Could you check a few things on this model? Use its own coordinates, in mm. Face numbers are marked on the shaded views. A direction names the side the tool comes from. Round coordinates to 2 decimals unless told otherwise and drop trailing zeros. Write each loop counter-clockwise with the first axis right and the second up, starting at its lowest first coordinate (ties: lowest second). Pieces come first, ordered by that corner, then holes. Notation, with made-up numbers: (38.25, 87) -> (91.25, 87) arc R24 ccw to (91.25, 102) -> close; hole circle Ø11 at (-16, 45.5). An arc over 180 degrees is marked (long way). Return JSON: item names as keys, results as strings.
from build123d import *

# Parameters (mm, degrees)
F1_DEPTH = 5
F2_DEPTH = 40
F3_DEPTH = 30


with BuildPart() as f1:
    # F0 (on Front) → F1 (new body)
    with BuildSketch(Plane.XZ):
        with BuildLine():
            Line((-22.0933434024, -7.5), (-27.3651991933, -7.5))
            ThreePointArc((-27.3651991933, -7.5), (-24.7292712978, -7.9784699581), (-22.0933434024, -7.5))
        make_face()
        with BuildLine():
            Line((27.7367906295, -7.5), (22.4649348386, -7.5))
            ThreePointArc((22.4649348386, -7.5), (25.1008627341, -7.9784699581), (27.7367906295, -7.5))
        make_face()
        with BuildLine():
            Line((32.5, -7.5), (32.5, -1.7043442256))
            ThreePointArc((32.5, -1.7043442256), (30.8950874158, -5.2405031728), (27.7367906295, -7.5))
            Line((27.7367906295, -7.5), (32.5, -7.5))
        make_face()
        with BuildLine():
            ThreePointArc((32.6008627341, -0.4784699581), (32.5756045187, 0.1365383775), (32.5, 0.7474043095))
            Line((32.5, 0.7474043095), (32.5, -1.7043442256))
            ThreePointArc((32.5, -1.7043442256), (32.5756045187, -1.0934782936), (32.6008627341, -0.4784699581))
        make_face()
        with BuildLine():
            Line((32.5, 7.5), (6.6143782777, 7.5))
            ThreePointArc((6.6143782777, 7.5), (9.1143782777, 4.1143782777), (10, 0))
            ThreePointArc((10, 0), (9.1143782777, -4.1143782777), (6.6143782777, -7.5))
            Line((6.6143782777, -7.5), (22.4649348386, -7.5))
            ThreePointArc((22.4649348386, -7.5), (20.3388295194, 5.3157547236), (32.5, 0.7474043095))
            Line((32.5, 0.7474043095), (32.5, 7.5))
        make_face()
        with BuildLine():
            Line((6.6143782777, 7.5), (-6.6143782777, 7.5))
            ThreePointArc((-6.6143782777, 7.5), (-10, 0), (-6.6143782777, -7.5))
            Line((-6.6143782777, -7.5), (-2.2328131871, -7.5))
            ThreePointArc((-2.2328131871, -7.5), (-4.1794324094, 5.698071659), (7.6857957181, -0.4006809507))
            ThreePointArc((7.6857957181, -0.4006809507), (6.2845483278, -4.7659090782), (2.6044046233, -7.5))
            Line((2.6044046233, -7.5), (6.6143782777, -7.5))
            ThreePointArc((6.6143782777, -7.5), (9.1143782777, -4.1143782777), (10, 0))
            ThreePointArc((10, 0), (9.1143782777, 4.1143782777), (6.6143782777, 7.5))
        make_face()
        with BuildLine():
            Line((-6.6143782777, 7.5), (-32.5, 7.5))
            Line((-32.5, 7.5), (-32.5, -7.5))
            Line((-32.5, -7.5), (-27.3651991933, -7.5))
            ThreePointArc((-27.3651991933, -7.5), (-29.0001342542, 5.6867331698), (-17.2292712978, -0.4784699581))
            ThreePointArc((-17.2292712978, -0.4784699581), (-18.56406817, -4.7493329144), (-22.0933434024, -7.5))
            Line((-22.0933434024, -7.5), (-6.6143782777, -7.5))
            ThreePointArc((-6.6143782777, -7.5), (-10, 0), (-6.6143782777, 7.5))
        make_face()
        with BuildLine():
            ThreePointArc((7.6857957181, -0.4006809507), (-4.1794324094, 5.698071659), (-2.2328131871, -7.5))
            Line((-2.2328131871, -7.5), (2.6044046233, -7.5))
            ThreePointArc((2.6044046233, -7.5), (6.2845483278, -4.7659090782), (7.6857957181, -0.4006809507))
        make_face()
        with BuildLine():
            ThreePointArc((-17.2292712978, -0.4784699581), (-29.0001342542, 5.6867331698), (-27.3651991933, -7.5))
            Line((-27.3651991933, -7.5), (-22.0933434024, -7.5))
            ThreePointArc((-22.0933434024, -7.5), (-18.56406817, -4.7493329144), (-17.2292712978, -0.4784699581))
        make_face()
        with BuildLine():
            Line((32.5, -1.7043442256), (32.5, 0.7474043095))
            ThreePointArc((32.5, 0.7474043095), (20.3388295194, 5.3157547236), (22.4649348386, -7.5))
            Line((22.4649348386, -7.5), (27.7367906295, -7.5))
            ThreePointArc((27.7367906295, -7.5), (30.8950874158, -5.2405031728), (32.5, -1.7043442256))
        make_face()
    extrude(amount=F1_DEPTH)

    # F0 (on Front) → F2 (join)
    with BuildSketch(Plane.XZ):
        with BuildLine():
            ThreePointArc((7.6857957181, -0.4006809507), (-4.1794324094, 5.698071659), (-2.2328131871, -7.5))
            Line((-2.2328131871, -7.5), (2.6044046233, -7.5))
            ThreePointArc((2.6044046233, -7.5), (6.2845483278, -4.7659090782), (7.6857957181, -0.4006809507))
        make_face()
        with BuildLine():
            ThreePointArc((6.6143782777, 7.5), (0, 10), (-6.6143782777, 7.5))
            Line((-6.6143782777, 7.5), (6.6143782777, 7.5))
        make_face()
        with BuildLine():
            Line((-2.2328131871, -7.5), (-6.6143782777, -7.5))
            ThreePointArc((-6.6143782777, -7.5), (0, -10), (6.6143782777, -7.5))
            Line((6.6143782777, -7.5), (2.6044046233, -7.5))
            ThreePointArc((2.6044046233, -7.5), (0.1857957181, -7.9006809507), (-2.2328131871, -7.5))
        make_face()
        with BuildLine():
            Line((6.6143782777, 7.5), (-6.6143782777, 7.5))
            ThreePointArc((-6.6143782777, 7.5), (-10, 0), (-6.6143782777, -7.5))
            Line((-6.6143782777, -7.5), (-2.2328131871, -7.5))
            ThreePointArc((-2.2328131871, -7.5), (-4.1794324094, 5.698071659), (7.6857957181, -0.4006809507))
            ThreePointArc((7.6857957181, -0.4006809507), (6.2845483278, -4.7659090782), (2.6044046233, -7.5))
            Line((2.6044046233, -7.5), (6.6143782777, -7.5))
            ThreePointArc((6.6143782777, -7.5), (9.1143782777, -4.1143782777), (10, 0))
            ThreePointArc((10, 0), (9.1143782777, 4.1143782777), (6.6143782777, 7.5))
        make_face()
    extrude(amount=F2_DEPTH)

    # F0 (on Front) → F3 (join)
    with BuildSketch(Plane.XZ):
        with BuildLine():
            Line((32.5, -1.7043442256), (32.5, 0.7474043095))
            ThreePointArc((32.5, 0.7474043095), (20.3388295194, 5.3157547236), (22.4649348386, -7.5))
            Line((22.4649348386, -7.5), (27.7367906295, -7.5))
            ThreePointArc((27.7367906295, -7.5), (30.8950874158, -5.2405031728), (32.5, -1.7043442256))
        make_face()
        with BuildLine():
            ThreePointArc((-17.2292712978, -0.4784699581), (-29.0001342542, 5.6867331698), (-27.3651991933, -7.5))
            Line((-27.3651991933, -7.5), (-22.0933434024, -7.5))
            ThreePointArc((-22.0933434024, -7.5), (-18.56406817, -4.7493329144), (-17.2292712978, -0.4784699581))
        make_face()
        with BuildLine():
            ThreePointArc((7.6857957181, -0.4006809507), (-4.1794324094, 5.698071659), (-2.2328131871, -7.5))
            Line((-2.2328131871, -7.5), (2.6044046233, -7.5))
            ThreePointArc((2.6044046233, -7.5), (6.2845483278, -4.7659090782), (7.6857957181, -0.4006809507))
        make_face()
    extrude(amount=-F3_DEPTH)


solid = f1.part
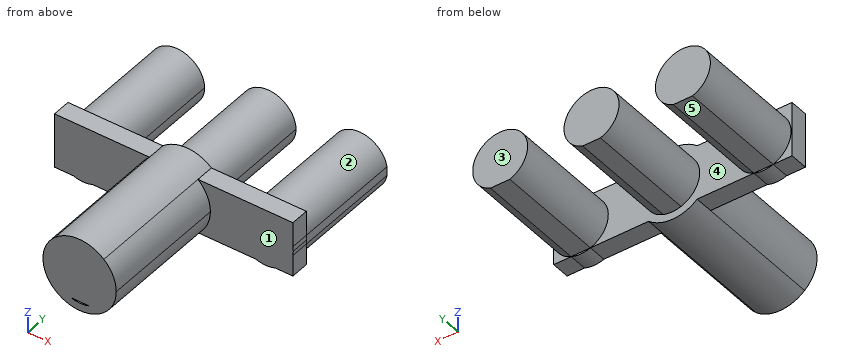
1) I want a section at A-A, the plane y = 4. Please give me the cut outline in (x, z), and give its area (3 significant figures).
Return value:
{"outline": "(-27.37, -7.5) -> (-22.09, -7.5) arc R7.5 ccw (long way) to start; (-2.23, -7.5) -> (2.6, -7.5) arc R7.5 ccw (long way) to start; (22.46, -7.5) -> (27.74, -7.5) arc R7.5 ccw to (32.5, -1.7) -> (32.5, 0.75) arc R7.5 ccw (long way) to start", "area": "525 mm²"}
2) Thinking about a two-plate mould opening in X: for the marked faces 1 and 2, which applies, pulls with the +X half, pulls with the -X half, needs draft (parallel to the pull), parting line crosses it, or undercut?
Return value:
{"face 1": "needs draft", "face 2": "undercut"}
3) Will these pins go through, and if not, where does the flat tip stop? pin 1 Ø1.5 at (x, y) = (15.5, -1.5) entering from +Z; pin 2 Ø2 at (y, z) = (13.5, -0.5) entering from +X; pin 3 Ø5 at (x, y) = (-7, -2) entering from -Z; pin 4 Ø10 at (x, z) = (10, 3) entering from -Y.
Return value:
{"pin 1": "z = 7.5", "pin 2": "x = 32.5", "pin 3": "z = -8.93", "pin 4": "y = -40"}
4) I want a section at D-D, the plane z = 4. Please give me the cut outline in (x, y).
Return value:
{"outline": "(-32.5, -5) -> (-9.17, -5) -> (-9.17, -40) -> (9.17, -40) -> (9.17, -5) -> (32.5, -5) -> (32.5, 0) -> (31.12, 0) -> (31.12, 30) -> (19.08, 30) -> (19.08, 0) -> (6.26, 0) -> (6.26, 30) -> (-5.89, 30) -> (-5.89, 0) -> (-18.71, 0) -> (-18.71, 30) -> (-30.75, 30) -> (-30.75, 0) -> (-32.5, 0) -> close"}
5) I want a section at C-C, the plane z = -2.5. Please give me the cut outline in (x, y).
Return value:
{"outline": "(-32.5, -5) -> (-9.68, -5) -> (-9.68, -40) -> (9.68, -40) -> (9.68, -5) -> (32.5, -5) -> (32.5, 0) -> (32.32, 0) -> (32.32, 30) -> (17.88, 30) -> (17.88, 0) -> (7.39, 0) -> (7.39, 30) -> (-7.01, 30) -> (-7.01, 0) -> (-17.51, 0) -> (-17.51, 30) -> (-31.95, 30) -> (-31.95, 0) -> (-32.5, 0) -> close"}
6) If I drill on probe 1 along X at (y, z) = (19, 3); probe 2 along X at (y, z) = (13, 2.75); probe 3 along Y at (x, z) = (9, -4.25), over which ranges is the centre line in solid material (lowest first)? Write a range as [from, to].
Return value:
{"probe 1": "[-31.37, -18.08], [-6.5, 6.87], [18.46, 31.75]", "probe 2": "[-31.5, -17.96], [-6.62, 6.99], [18.33, 31.87]", "probe 3": "[-40, 0]"}
7) For the marked faces 3, 4 and 5, which set-ups out of +Z, -Z, +X, -X, +Y, -Y let a thin tool reach every point of the face, with its end or its side?
Return value:
{"face 3": "+Z, -Z, +X, -X, +Y", "face 4": "+Y", "face 5": "-Z, +X, -X, +Y"}
8) I want a section at B-B, the plane y = -7. Please give me the cut outline in (x, z), and give its area (3 significant figures).
Return value:
{"outline": "circle Ø20 at (0, 0); hole (-2.23, -7.5) arc R7.5 ccw to (2.6, -7.5) -> close", "area": "313 mm²"}
